Build history of the part. All positions in model axes, mm. Face numbers are marked on the shaded views. A direction names the side the tool comes from. Give positions to 0.01 mm unless a question says otherwise; leave off trailing zeros. Loops run counter-clockwise (first coordinate to the right, second up) from the corner with the lowest first, then second, coordinate; pieces in that order, holes last.
1) Band-saw the part on C-C on z = 24.5. List the corners of the cut face in (x, y).
2) Wall check: line 1 (Z direction, x = -10, y = 1.75); line 2 (Y direction, x = 5, z = 26.5); line 3 (Z direction, x = 16.5, y = -0.75). Give the ranges that are in metal, low to high.
3) Band-saw the part on D-D on y = -4.5. List the corners of the cut face in (x, z), then the cut area to 3 significant figures.
4) Band-saw the part on B-B on x = 0. List the corners of the cut face in (y, z).
5) 3-axis set-ups, long thin cutter, end or side, ignore diameter. For the marked faces 1 and 2: which of +Z, -Z, +X, -X, +Y, -Y reach the whole face in a straight line?
6) Band-saw the part on A-A on y = 0. List the corners of the cut face in (x, z), then the cut area to 3 significant figures.
7) Flat gauge pins, fed straight in: P1, Ø4, axis at y = -1, z = 20, coming from the -X side; P2, Ø2, axis at x = -12.5, y = 1.5, coming from the -Z side. Where does each tip first touch, or does it go through?
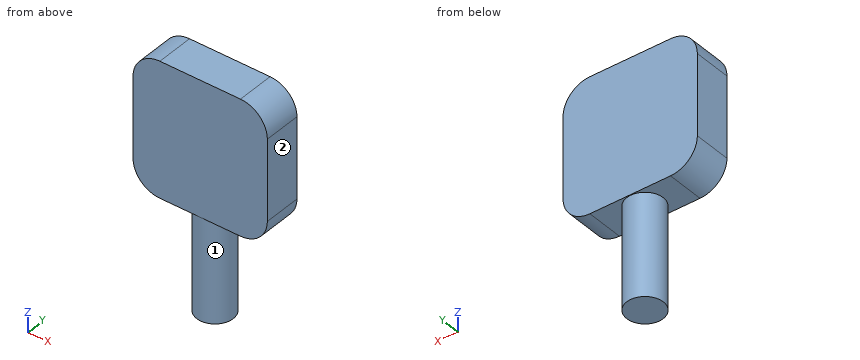
```python
from build123d import *

# Parameters (mm, degrees)
BOSS_EXTRUDE1_DEPTH      = 73
BOSS_EXTRUDE1_DEPTH_BACK = 10
SKETCH1_R                = 6.75
BOSS_EXTRUDE2_DEPTH      = 7
BOSS_EXTRUDE2_DEPTH_BACK = 7


with BuildPart() as part:
    # Sketch1 → Boss-Extrude1 (new, two sides: drawn at the far end of the back side and taken through both)
    with BuildSketch(Plane.XY.offset(-BOSS_EXTRUDE1_DEPTH_BACK)):
        Circle(SKETCH1_R)
    extrude(amount=BOSS_EXTRUDE1_DEPTH + BOSS_EXTRUDE1_DEPTH_BACK)

    # Sketch2 → Boss-Extrude2 (add, two sides: drawn at the far end of the back side and taken through both)
    with BuildSketch(Plane(origin=(0, 0, 0), x_dir=(1, 0, 0), z_dir=(0, 1, 0)).offset(-BOSS_EXTRUDE2_DEPTH_BACK)):
        with BuildLine():
            Line((-15, -78), (15, -78))
            ThreePointArc((15, -78), (22.071067812, -75.071067812), (25, -68))
            Line((25, -68), (25, -38))
            ThreePointArc((25, -38), (22.071067812, -30.928932188), (15, -28))
            Line((15, -28), (-15, -28))
            ThreePointArc((-15, -28), (-22.071067812, -30.928932188), (-25, -38))
            Line((-25, -38), (-25, -68))
            ThreePointArc((-25, -68), (-22.071067812, -75.071067812), (-15, -78))
        make_face()
    extrude(amount=BOSS_EXTRUDE2_DEPTH + BOSS_EXTRUDE2_DEPTH_BACK)


solid = part.part
```
Findings below:
1. outline: circle Ø13.5 at (0, 0)
2. line 1: z = 28 to 78
2. line 2: y = -4.53 to 4.53
2. line 3: z = 28.11 to 77.89
3. outline: (-25, 38) arc R10 ccw to (-15, 28) - (-5.03, 28) - (-5.03, -10) - (5.03, -10) - (5.03, 28) - (15, 28) arc R10 ccw to (25, 38) - (25, 68) arc R10 ccw to (15, 78) - (-15, 78) arc R10 ccw to (-25, 68) - close
3. area: 2,800 mm2
4. outline: (-7, 28) - (-6.75, 28) - (-6.75, -10) - (6.75, -10) - (6.75, 28) - (7, 28) - (7, 78) - (-7, 78) - close
5. face 1: -Z
5. face 2: +Z, -Z, +X, +Y, -Y
6. outline: (-25, 38) arc R10 ccw to (-15, 28) - (-6.75, 28) - (-6.75, -10) - (6.75, -10) - (6.75, 28) - (15, 28) arc R10 ccw to (25, 38) - (25, 68) arc R10 ccw to (15, 78) - (-15, 78) arc R10 ccw to (-25, 68) - close
6. area: 2,930 mm2
7. P1: stops at x = -6.75
7. P2: stops at z = 28
